```python
from build123d import *

# Parameters (mm, degrees)
BOSS_EXTRUDE1_DEPTH                                 = 25.4
FILLET1_R                                           = 3.937
FILLET2_R                                           = 7.9375
F_5_16_CLEARANCE_HOLE1_D                            = 8.4328
CSK_FOR_5_16_FLAT_HEAD_MACHINE_SCREW_10_D           = 8.4328
CSK_FOR_5_16_FLAT_HEAD_MACHINE_SCREW_10_CSINK_D     = 16.129
CSK_FOR_5_16_FLAT_HEAD_MACHINE_SCREW_10_CSINK_ANGLE = 100
CUT_EXTRUDE2_DEPTH                                  = 19.05


with BuildPart() as part:
    # Sketch2 → Boss-Extrude1 (new body)
    with BuildSketch(Plane(origin=(0, 0, 0), x_dir=(1, 0, 0), z_dir=(0, 1, 0))):
        Polygon((-11.811, 17.4625), (-3.937, 17.4625), (-3.937, 28.575), (3.937, 28.575), (3.937, 17.4625), (11.811, 17.4625), (11.811, 28.575), (34.925, 28.575), (34.925, -6.35), (22.225, -15.875), (-22.225, -15.875), (-34.925, -6.35), (-34.925, 28.575), (-11.811, 28.575), align=None)
    extrude(amount=BOSS_EXTRUDE1_DEPTH)

    # Fillet1
    fillet1_edges = [part.edges().sort_by_distance(p)[0] for p in [
        (11.811, 12.7, -17.4625),
        (3.937, 12.7, -17.4625),
        (3.937, 12.7, -28.575),
        (-3.937, 12.7, -28.575),
        (-3.937, 12.7, -17.4625),
        (-11.811, 12.7, -17.4625),
    ]]
    fillet(fillet1_edges, radius=FILLET1_R - 0.0001)  # a hair under: the kernel refuses the full size

    # Fillet2
    fillet2_edges = [part.edges().sort_by_distance(p)[0] for p in [
        (34.925, 12.7, 6.35),
        (22.225, 12.7, 15.875),
        (-22.225, 12.7, 15.875),
        (-34.925, 12.7, 6.35),
        (34.925, 12.7, -28.575),
        (11.811, 12.7, -28.575),
        (-11.811, 12.7, -28.575),
        (-34.925, 12.7, -28.575),
    ]]
    fillet(fillet2_edges, radius=FILLET2_R)

    # 5/16 Clearance Hole1 (through all)
    with Locations(Plane(origin=(0, 25.4, 0), x_dir=(1, 0, 0), z_dir=(0, 1, 0))):
        with Locations((-23.8252, 19.05), (23.7998, 19.05)):
            Hole(F_5_16_CLEARANCE_HOLE1_D / 2)

    # CSK for 5/16 Flat Head Machine Screw (100)1 (through all)
    with Locations(Plane(origin=(0, 0, 0), x_dir=(-1, 0, 0), z_dir=(0, -1, 0))):
        with Locations((-23.8125, 0), (23.8125, 0)):
            CounterSinkHole(CSK_FOR_5_16_FLAT_HEAD_MACHINE_SCREW_10_D / 2, CSK_FOR_5_16_FLAT_HEAD_MACHINE_SCREW_10_CSINK_D / 2, counter_sink_angle=CSK_FOR_5_16_FLAT_HEAD_MACHINE_SCREW_10_CSINK_ANGLE)

    # Sketch8 → Cut-Extrude2 (cut)
    with BuildSketch(Plane(origin=(0, 25.4, 0), x_dir=(1, 0, 0), z_dir=(0, 1, 0))):
        with BuildLine():
            Line((24.341666667, -14.2875), (31.75, -8.73125))
            ThreePointArc((31.75, -8.73125), (34.087015829, -5.931007914), (34.925, -2.38125))
            Line((34.925, -2.38125), (34.925, 20.6375))
            ThreePointArc((34.925, 20.6375), (32.600160076, 15.024839924), (26.9875, 12.7))
            ThreePointArc((26.9875, 12.7), (0, 17.4625), (-26.9875, 12.7))
            ThreePointArc((-26.9875, 12.7), (-32.600160076, 15.024839924), (-34.925, 20.6375))
            Line((-34.925, 20.6375), (-34.925, -2.38125))
            ThreePointArc((-34.925, -2.38125), (-34.087015829, -5.931007914), (-31.75, -8.73125))
            Line((-31.75, -8.73125), (-24.341666667, -14.2875))
            ThreePointArc((-24.341666667, -14.2875), (-22.089224559, -15.467673678), (-19.579166667, -15.875))
            Line((-19.579166667, -15.875), (19.579166667, -15.875))
            ThreePointArc((19.579166667, -15.875), (22.089224559, -15.467673678), (24.341666667, -14.2875))
        make_face()
    extrude(amount=-CUT_EXTRUDE2_DEPTH, mode=Mode.SUBTRACT)


solid = part.part
```
Check sheet for the modelled part. Datum: model origin and axes. Units: mm. A direction names the side the tool comes from. Round coordinates to 2 decimals unless told otherwise and drop trailing zeros. Write each loop counter-clockwise with the first axis right and the second up, starting at its lowest first coordinate (ties: lowest second). Pieces come first, ordered by that corner, then holes. Notation, with made-up numbers: (42, 53.5) -> (55, 53.5) arc R13 ccw to (55, 65.5) -> close; hole circle Ø3 at (4, -8). An arc over 180 degrees is marked (long way). Put each result on its own line as item: value.
(1) Sectioned sample at B-B (y = 13.25). Count the separate pieces of the cut face and the enclosed holes in it, plus the area to 3 significant figures.
Values found:
separate pieces: 1
enclosed holes: 2
area: 576 mm^2
(2) Sectioned sample at C-C (z = -19.05). Enter the section's corners in (x, y) (3 decimals).
Values found:
outline: (-34.925, 0) -> (-28.042, 0) -> (-28.042, 25.4) -> (-34.765, 25.4) -> (-34.765, 6.35) -> (-34.925, 6.35) -> close; (-19.609, 0) -> (-11.033, 0) -> (-11.033, 25.4) -> (-19.609, 25.4) -> close; (-4.715, 0) -> (4.715, 0) -> (4.715, 25.4) -> (-4.715, 25.4) -> close; (11.033, 0) -> (19.583, 0) -> (19.583, 25.4) -> (11.033, 25.4) -> close; (28.016, 0) -> (34.925, 0) -> (34.925, 6.35) -> (34.765, 6.35) -> (34.765, 25.4) -> (28.016, 25.4) -> close
(3) Tool access check on faces 4 (the face through (5.06, 12.878, -18.646)), 5 (the face through (-19.918, 4.811, 1.615)), 6 (the face through (0.39, 16.01, -17.46)). Record the directions out of +Z, -Z, +X, -X, +Y, -Y that give a thin tool (end or side, any length) a straight path to the whole face; none if there is none.
Values found:
face 4: -Z, +Y, -Y
face 5: +Y, -Y
face 6: +Z, +Y
(4) Mould release check, pull along X, two halves, no side actions. Record for faces 1 (the face through (34.925, 3, -9)), 2 (the face through (-5.121, 12.878, -18.585)), 3 (the face through (23, 13, -28.575)): released by +X, released by -X, zero draft, split by the parting line, or undercut.
Values found:
face 1: released by +X
face 2: undercut
face 3: zero draft
(5) Go/stop test with flat-tipped pins: pin 1 Ø11 at (x, z) = (-23.81, 0) entering from +Y; pin 2 Ø10 at (x, y) = (-2, 13.5) entering from +Z; pin 3 Ø3.5 at (y, z) = (13, -23.5) entering from -X; pin 4 Ø6.5 at (x, z) = (23.81, 0) entering from -Y. Record where each tip stops, or that it passes through.
Values found:
pin 1: stops at y = 6.35
pin 2: stops at z = -17.15
pin 3: stops at x = -34.85
pin 4: passes through
(6) Material ranges on line 1 (X direction, y = 8, z = -19.05); line 2 (Y direction, x = 4, z = 5); line 3 (Z direction, x = 7.5, y = 4.75) (3 decimals), recorded low to high.
Values found:
line 1: x = -34.76 to -28.04, -19.61 to -11.03, -4.71 to 4.71, 11.03 to 19.58, 28.02 to 34.76
line 2: y = 0 to 6.35
line 3: z = -17.48 to 15.875
(7) Sectioned sample at A-A (z = 0). Enter the section's corners in (x, y) (3 decimals).
Values found:
outline: (-34.925, 0) -> (-31.877, 0) -> (-28.029, 3.229) -> (-28.029, 6.35) -> (-34.925, 6.35) -> close; (-19.596, 3.229) -> (-15.748, 0) -> (15.748, 0) -> (19.596, 3.229) -> (19.596, 6.35) -> (-19.596, 6.35) -> close; (28.029, 3.229) -> (31.877, 0) -> (34.925, 0) -> (34.925, 6.35) -> (28.029, 6.35) -> close
